```python
from build123d import *

# Parameters (mm, degrees)
F0_W     = 300
F0_H     = 200
F1_DEPTH = 5


with BuildPart() as f1:
    # F0 (on Top) → F1 (new body)
    with BuildSketch(Plane.XY):
        Rectangle(F0_W, F0_H)
        with BuildLine():
            ThreePointArc((98.964391, -70), (92, -77.705161), (85.035609, -70))
            Line((85.035609, -70), (85.035609, 70))
            ThreePointArc((85.035609, 70), (92, 77.705161), (98.964391, 70))
            Line((98.964391, 70), (98.964391, -70))
        make_face(mode=Mode.SUBTRACT)
        with BuildLine():
            Line((-85.035609, 70), (-85.035609, -70))
            ThreePointArc((-85.035609, -70), (-92, -77.705161), (-98.964391, -70))
            Line((-98.964391, -70), (-98.964391, 70))
            ThreePointArc((-98.964391, 70), (-92, 77.705161), (-85.035609, 70))
        make_face(mode=Mode.SUBTRACT)
    extrude(amount=F1_DEPTH)


solid = f1.part
```
Can you work these out from the model? Positions are in its coordinate system, mm. Round coordinates to 2 decimals unless told otherwise and drop trailing zeros. Loops run counter-clockwise (first coordinate to the right, second up) from the corner with the lowest first, then second, coordinate; pieces in that order, holes last. Notation, with made-up numbers: M 69.5,-21 L 105.5,-21 A11 cw 105.5,-1 Z; hole C -12.5,47.25 d6. An arc over 180 degrees is marked long. Write item = value, one per line. Start each with the question number.
(1) If we mould it in two halves opening along Y, with no side actions, what happens to faces 1 (the face through (-2, 1, 5)), 2 (the face through (92.164, -77.703, 2.465))? For each: released by +Y, released by -Y, zero draft, split by the parting line, or undercut.
(2) I'm going to push a flat-ended pin straight in: P1, Ø8.5, axis at x = -92, y = -70.71, coming from the -Z side. Where does the tip first touch, or does it pass through?
(3) Suppose I cut it at B-B on y = -25. Write out the boundary of the cut face in (x, z).
(4) Suppose I cut it at A-A on x = 92. Write out the boundary of the cut face in (y, z), plus the area to 3 significant figures.
(5) Suppose I cut it at C-C on z = 2.3. Write out the boundary of the cut face in (x, y).
(6) I need wall thicknesses on line 1 along X through (y, z) = (32.5, 0.55); line 2 along Y through (x, z) = (92, 1.5); line 3 along Y through (x, z) = (-93, 0.9). Which ranges of each line are inside material? Lowest first, please.
Answer block:
q1.face_1 = zero draft
q1.face_2 = undercut
q2.P1 = through
q3.outline = M -150,0 L -98.96,0 L -98.96,5 L -150,5 Z; M -85.04,0 L 85.04,0 L 85.04,5 L -85.04,5 Z; M 98.96,0 L 150,0 L 150,5 L 98.96,5 Z
q4.outline = M -100,0 L -77.71,0 L -77.71,5 L -100,5 Z; M 77.71,0 L 100,0 L 100,5 L 77.71,5 Z
q4.area = 223 mm²
q5.outline = M -150,-100 L 150,-100 L 150,100 L -150,100 Z; hole M -98.96,-70 A7 ccw long -85.04,-70 L -85.04,70 A7 ccw long -98.96,70 Z; hole M 85.04,-70 A7 ccw long 98.96,-70 L 98.96,70 A7 ccw long 85.04,70 Z
q6.line_1 = -150 to -98.96, -85.04 to 85.04, 98.96 to 150
q6.line_2 = -100 to -77.71, 77.71 to 100
q6.line_3 = -100 to -77.63, 77.63 to 100
